For this review, use the dimensioned drawing (mm, ordinates from the lowest corner) and the shaded views. Give positions to 0.01 mm unless a question says otherwise; leave off trailing zeros. Write each loop counter-clockwise with the first axis right and the second up, starting at its lowest first coordinate (ties: lowest second). Pieces come first, ordered by that corner, then holes. Notation, with made-up numbers: M 28,67 L 84,67 A8 cw 84,81 Z; hole C -22.5,-7.75 d4. An arc over 180 degrees is marked long. Answer in a Markdown table with one row per item.
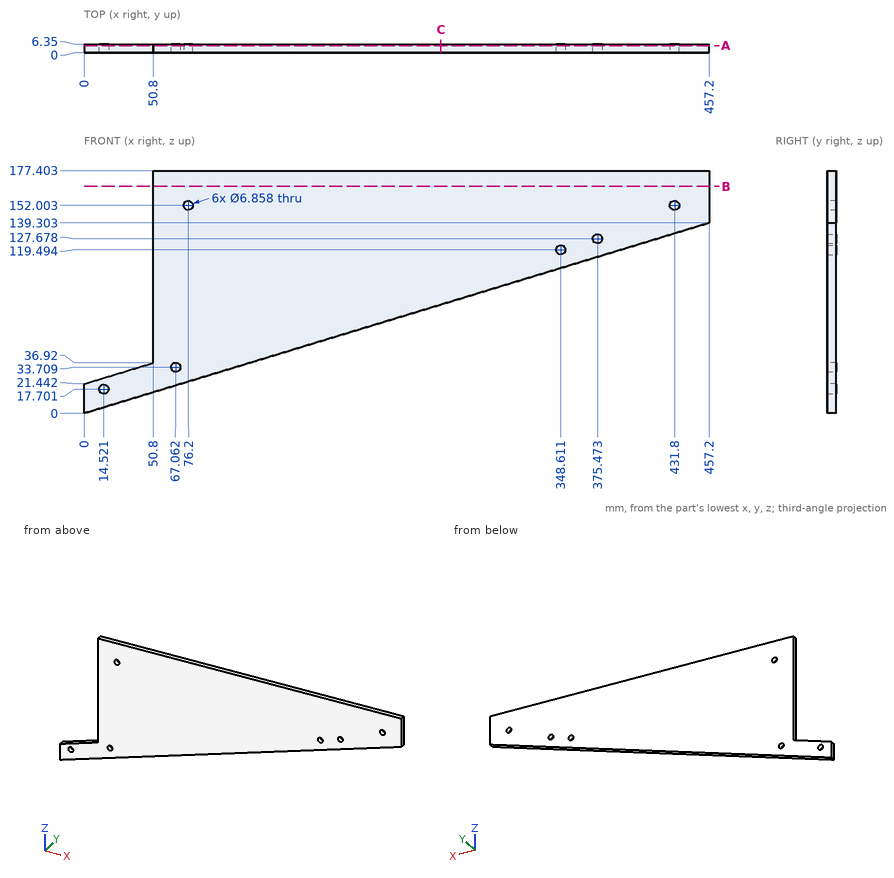
1) Add section C-C (x = 261). Write out the cut boundary in (y, z).
Geometry says:
| item | result |
|---|---|
| outline | M 0,79.52 L 6.35,79.52 L 6.35,177.4 L 0,177.4 Z |
2) Add section A-A (y = 5.25). Write out the cut boundary in (x, z).
Geometry says:
| item | result |
|---|---|
| outline | M 0,0 L 457.2,139.3 L 457.2,177.4 L 50.8,177.4 L 50.8,36.92 L 0,21.44 Z; hole C 14.52,17.7 d6.86; hole C 67.06,33.71 d6.86; hole C 76.2,152 d6.86; hole C 348.61,119.49 d6.86; hole C 375.47,127.68 d6.86; hole C 431.8,152 d6.86 |
3) To check wall thickness, follow probe 1 along X at (y, z) = (4.25, 167); probe 2 along Z at (x, y) = (211.5, 1.25); probe 3 along Z at (x, y) = (86, 5.5). State the ranges of each line that lie inside material, in increasing order. Write a range as [from, to].
Geometry says:
| item | result |
|---|---|
| probe 1 | [50.8, 457.2] |
| probe 2 | [64.44, 177.4] |
| probe 3 | [26.2, 177.4] |
4) Insertion check: P1, Ø1.9, axis at y = 4, z = 99.5, coming from the -X side; P2, Ø5.5, axis at x = 76.2, z = 152, coming from the -Y side. Each pin has a flat end and moves straight along its axis. Give the tip position at first contact, or say it passes through.
Geometry says:
| item | result |
|---|---|
| P1 | x = 50.8 |
| P2 | through |
5) Add section B-B (z = 166). Write out the cut boundary in (x, y), and give its area (3 significant figures).
Geometry says:
| item | result |
|---|---|
| outline | M 50.8,0 L 457.2,0 L 457.2,6.35 L 50.8,6.35 Z |
| area | 2,580 mm^2 |
